The listing builds one solid part. Answer for the finished solid, in the listing's coordinates (mm). A direction names the side the tool comes from. Give positions to 0.01 mm unless a question says otherwise; leave off trailing zeros. Loops run counter-clockwise (first coordinate to the right, second up) from the corner with the lowest first, then second, coordinate; pieces in that order, holes last. Notation, with made-up numbers: (-3.5, 2.5) - (12.5, 2.5) arc R13 cw to (12.5, 12.5) - close; hole circle Ø6 at (-40, 41). An arc over 180 degrees is marked (long way). Write item = value, one per line. Start each with the question number.
1) Flat-ended cylindrical pins translate along their axes: P1, Ø4, axis at x = 8.5, y = -11.5, coming from the +Z side; P2, Ø4, axis at x = 11, y = 8, coming from the +Z side; P3, Ø12, axis at x = 16, y = -8, coming from the -Z side. Find the tip coordinate at first contact, or state that the pin passes through.
2) Which of the six approach directions +Z, -Z, +X, -X, +Y, -Y give full straight-line access (tool end or side, diameter ignored) to faces 1 (the cylindrical face through (-0.976, 11.744, -7.436)), 2 (the cylindrical face through (6.93, -11.48, 2.87)), 3 (the cylindrical face through (11.744, 0.33, 7.493))?
3) The part is cut by section B-B on x = -12. Write down the section's boundary in (y, z).
4) Consider probe 1 along Y at (x, z) = (-15.5, -4); probe 2 along Y at (x, z) = (-8, 2.25); probe 3 along Z at (x, y) = (-12.5, 6). Determine where each line is inside the solid, lowest interval first.
5) The part is cut by section A-A on z = 0. Write down the section's boundary in (x, y), plus the area to 3 significant figures.
from build123d import *

# Parameters (mm, degrees)
SKETCH1_R           = 7.5
BOSS_EXTRUDE1_DEPTH = 20
SKETCH2_R           = 7.5
BOSS_EXTRUDE2_DEPTH = 20
FILLET1_R           = 1


with BuildPart() as part:
    # Sketch1 → Boss-Extrude1 (new body, symmetric)
    with BuildSketch(Plane(origin=(0, 0, 0), x_dir=(1, 0, 0), z_dir=(0, 1, 0))):
        Circle(SKETCH1_R)
    extrude(amount=BOSS_EXTRUDE1_DEPTH, both=True)

    # Sketch2 → Boss-Extrude2 (add, symmetric)
    with BuildSketch(Plane(origin=(0, 0, 0), x_dir=(0, 0, -1), z_dir=(1, 0, 0))):
        Circle(SKETCH2_R)
    extrude(amount=BOSS_EXTRUDE2_DEPTH, both=True)

    # Fillet1
    fillet1_edges = [part.edges().sort_by_distance(p)[0] for p in [
        (-7.5, -20, 0),
        (-7.5, 20, 0),
        (-20, 0, 7.5),
        (20, 0, 7.5),
    ]]
    fillet(fillet1_edges, radius=FILLET1_R)


solid = part.part
Answer below:
q1.P1 = 3.74
q1.P2 = 4.5
q1.P3 = -7.23
q2.face_1 = +Y
q2.face_2 = -Y
q2.face_3 = +X
q3.outline = circle Ø15 at (0, 0)
q4.probe_1 = -6.34 to 6.34
q4.probe_2 = -7.15 to 7.15
q4.probe_3 = -4.5 to 4.5
q5.outline = (-20, -6.5) arc R1 ccw to (-19, -7.5) - (-7.5, -7.5) - (-7.5, -19) arc R1 ccw to (-6.5, -20) - (6.5, -20) arc R1 ccw to (7.5, -19) - (7.5, -7.5) - (19, -7.5) arc R1 ccw to (20, -6.5) - (20, 6.5) arc R1 ccw to (19, 7.5) - (7.5, 7.5) - (7.5, 19) arc R1 ccw to (6.5, 20) - (-6.5, 20) arc R1 ccw to (-7.5, 19) - (-7.5, 7.5) - (-19, 7.5) arc R1 ccw to (-20, 6.5) - close
q5.area = 973 mm2
